The listing builds one solid part. Answer for the finished solid, in the listing's coordinates (mm). Face numbers are marked on the shaded views. A direction names the side the tool comes from. Give positions to 0.01 mm unless a question says otherwise; leave off trailing zeros. Order: outer loops, then holes, each group sorted by start corner. A loop starts at its lowest first (then second) coordinate and runs counter-clockwise, first axis right, second up. Notation, with made-up numbers: (58.5, 87.5) - (83.5, 87.5) arc R11 cw to (83.5, 108.5) - close; hole circle Ø11 at (48.25, 82.5). An arc over 180 degrees is marked (long way). Write each question's results on one line, items separated by ' | '. Start each with the question number.
1. A flat-ended cylindrical pin translates along its axis: pin 1 (15 mm diameter, centred on x = 22.225, y = 38.1, fed in from -Z). Find the tip coordinate at first contact, or state that the pin passes through.
2. Section C-C (z = 10) is taken. Give the vertices of the cut face in (x, y) (1 decimal), and give its area (3 significant figures).
3. Determine the mould class of the marked faces 1, 2, 3 and 4 for opening direction X: released by +X, released by -X, zero draft, split by the parting line, or undercut.
4. Find the intervals of material crossed by L1, parallel to Y at x = -70.5, z = 3; L2, parallel to X at y = -90, z = 6.5; L3, parallel to Y at x = 44, z = 42.5, in increasing order.
5. Section A-A (y = 38.1) is taken. State how many separate pieces and enclosed holes the cut face has, and give its area (3 significant figures).
6. Which of the six approach directions +Z, -Z, +X, -X, +Y, -Y give full straight-line access (tool end or side, diameter ignored) to the marked faces 5 and 6?
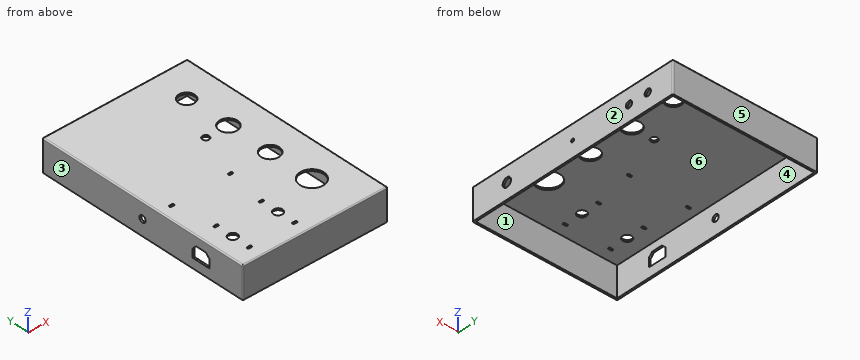
from build123d import *

# Parameters (mm, degrees)
F0_W      = 203.2
F0_H      = 304.8
F1_DEPTH  = 44.45
F2_T      = -2.54
F3_W      = 6.35
F3_H      = 3.175
F4_DEPTH  = 25.4
F5_R      = 1.58749
F7_D      = 33.3375
F7_DEPTH  = 19.05
F7_TIP    = 10.0155954434
F8_D      = 25.4
F8_DEPTH  = 19.05
F8_TIP    = 7.6309298617
F9_D      = 22.225
F9_DEPTH  = 19.05
F9_TIP    = 6.6770636289
F11_D     = 4.7625
F11_DEPTH = 19.05
F11_TIP   = 1.4307993491
F12_D     = 9.525
F12_DEPTH = 19.05
F12_TIP   = 2.8615986981
F13_D     = 12.7
F13_DEPTH = 19.05
F13_TIP   = 3.8154649308
F15_DEPTH = 25.4
F16_D     = 12.7
F16_DEPTH = 19.05
F16_TIP   = 3.8154649308
F17_W     = 6.35
F17_H     = 3.175
F18_DEPTH = 25.4
F19_R     = 1.58749
F20_D     = 9.525
F20_DEPTH = 5.715
F20_TIP   = 2.8615986981
F21_D     = 9.525
F21_DEPTH = 5.715
F21_TIP   = 2.8615986981
F22_R     = 1.5875


# Not quite as in the source:
# - a fillet or chamfer is up to 0.001 mm smaller than in the source, because OpenCascade refuses the exact size


with BuildPart() as f1:
    # F0 (on Top) → F1 (new body)
    with BuildSketch(Plane.XY):
        Rectangle(F0_W, F0_H)
    extrude(amount=F1_DEPTH)

    # F2
    f2_openings = [f1.faces().sort_by_distance(p)[0] for p in [
        (0, 0, 0),
    ]]
    offset(amount=F2_T, openings=f2_openings)

    # F3 (on face) → F4 (cut)
    with BuildSketch(Plane.XY.offset(44.45)):
        with Locations((-74.6125, -133.35)):
            Rectangle(F3_W, F3_H)
        with Locations((-74.6125, -82.55)):
            Rectangle(F3_W, F3_H)
        with Locations((-11.1125, -82.55)):
            Rectangle(F3_W, F3_H)
        with Locations((-11.1125, -133.35)):
            Rectangle(F3_W, F3_H)
    extrude(amount=-F4_DEPTH, mode=Mode.SUBTRACT)

    # F5 (radius 1.5875 in the source; OpenCascade refuses exactly that, so slightly less here)
    f5_edges = [f1.edges().sort_by_distance(p)[0] for p in [
        (-77.7875, -131.7625, 43.18),
        (-14.2875, -131.7625, 43.18),
        (-77.7875, -80.9625, 43.18),
        (-71.4375, -80.9625, 43.18),
        (-7.9375, -80.9625, 43.18),
        (-7.9375, -131.7625, 43.18),
        (-71.4375, -131.7625, 43.18),
        (-14.2875, -134.9375, 43.18),
        (-77.7875, -134.9375, 43.18),
        (-77.7875, -84.1375, 43.18),
        (-14.2875, -84.1375, 43.18),
        (-7.9375, -134.9375, 43.18),
        (-7.9375, -84.1375, 43.18),
        (-71.4375, -84.1375, 43.18),
        (-71.4375, -134.9375, 43.18),
        (-14.2875, -80.9625, 43.18),
    ]]
    fillet(f5_edges, radius=F5_R)

    # F7
    with Locations(Plane.XY.offset(44.45)):
        with Locations((53.975, -88.9)):
            Hole(F7_D / 2, depth=F7_DEPTH)
            with Locations((0, 0, -(F7_DEPTH + F7_TIP / 2))):  # 118° drill point
                Cone(0, F7_D / 2, F7_TIP, mode=Mode.SUBTRACT)

    # F8
    with Locations(Plane.XY.offset(44.45)):
        with Locations((53.975, -25.4), (53.975, 38.1)):
            Hole(F8_D / 2, depth=F8_DEPTH)
            with Locations((0, 0, -(F8_DEPTH + F8_TIP / 2))):  # 118° drill point
                Cone(0, F8_D / 2, F8_TIP, mode=Mode.SUBTRACT)

    # F9
    with Locations(Plane.XY.offset(44.45)):
        with Locations((53.975, 101.6)):
            Hole(F9_D / 2, depth=F9_DEPTH)
            with Locations((0, 0, -(F9_DEPTH + F9_TIP / 2))):  # 118° drill point
                Cone(0, F9_D / 2, F9_TIP, mode=Mode.SUBTRACT)

    # F11
    with Locations(Plane.YZ.offset(101.6)):
        with Locations((0, 22.225)):
            Hole(F11_D / 2, depth=F11_DEPTH)
            with Locations((0, 0, -(F11_DEPTH + F11_TIP / 2))):  # 118° drill point
                Cone(0, F11_D / 2, F11_TIP, mode=Mode.SUBTRACT)

    # F12
    with Locations(Plane.YZ.offset(101.6)):
        with Locations((85.725, 22.225), (114.3, 22.225)):
            Hole(F12_D / 2, depth=F12_DEPTH)
            with Locations((0, 0, -(F12_DEPTH + F12_TIP / 2))):  # 118° drill point
                Cone(0, F12_D / 2, F12_TIP, mode=Mode.SUBTRACT)

    # F13
    with Locations(Plane.YZ.offset(101.6)):
        with Locations((-100.0125, 22.225)):
            Hole(F13_D / 2, depth=F13_DEPTH)
            with Locations((0, 0, -(F13_DEPTH + F13_TIP / 2))):  # 118° drill point
                Cone(0, F13_D / 2, F13_TIP, mode=Mode.SUBTRACT)

    # F14 (on face) → F15 (cut)
    with BuildSketch(Plane(origin=(-101.6, 0, 0), x_dir=(0, -1, 0), z_dir=(-1, 0, 0))):
        Polygon((101.6, 25.5999010921), (96.2436510921, 30.95625), (81.5563489079, 30.95625), (76.2, 25.5999010921), (76.2, 18.8500989079), (81.5563489079, 13.49375), (96.2436510921, 13.49375), (101.6, 18.8500989079), align=None)
        Polygon((81.5563489079, 13.49375), (76.2, 18.8500989079), (76.2, 13.49375), align=None)
        Polygon((101.6, 13.49375), (101.6, 18.8500989079), (96.2436510921, 13.49375), align=None)
    extrude(amount=-F15_DEPTH, mode=Mode.SUBTRACT)

    # F16
    with Locations(Plane.XY.offset(44.45)):
        with Locations((-74.6125, -107.95), (-11.1125, -107.95)):
            Hole(F16_D / 2, depth=F16_DEPTH)
            with Locations((0, 0, -(F16_DEPTH + F16_TIP / 2))):  # 118° drill point
                Cone(0, F16_D / 2, F16_TIP, mode=Mode.SUBTRACT)

    # F17 (on face) → F18 (cut)
    with BuildSketch(Plane.XY.offset(44.45)):
        with Locations((-84.1375, -25.4)):
            Rectangle(F17_W, F17_H)
        with Locations((-1.5875, -25.4)):
            Rectangle(F17_W, F17_H)
    extrude(amount=-F18_DEPTH, mode=Mode.SUBTRACT)

    # F19 (radius 1.5875 in the source; OpenCascade refuses exactly that, so slightly less here)
    f19_edges = [f1.edges().sort_by_distance(p)[0] for p in [
        (-87.3125, -23.8125, 43.18),
        (-4.7625, -23.8125, 43.18),
        (-80.9625, -23.8125, 43.18),
        (1.5875, -23.8125, 43.18),
        (-87.3125, -26.9875, 43.18),
        (-4.7625, -26.9875, 43.18),
        (-80.9625, -26.9875, 43.18),
        (1.5875, -26.9875, 43.18),
    ]]
    fillet(f19_edges, radius=F19_R)

    # F20
    with Locations(Plane(origin=(-101.6, 0, 0), x_dir=(0, -1, 0), z_dir=(-1, 0, 0))):
        with Locations((0, 22.225)):
            Hole(F20_D / 2, depth=F20_DEPTH)
            with Locations((0, 0, -(F20_DEPTH + F20_TIP / 2))):  # 118° drill point
                Cone(0, F20_D / 2, F20_TIP, mode=Mode.SUBTRACT)

    # F21
    with Locations(Plane.XY.offset(44.45)):
        with Locations((22.225, 38.1)):
            Hole(F21_D / 2, depth=F21_DEPTH)
            with Locations((0, 0, -(F21_DEPTH + F21_TIP / 2))):  # 118° drill point
                Cone(0, F21_D / 2, F21_TIP, mode=Mode.SUBTRACT)

    # F22
    f22_edges = [f1.edges().sort_by_distance(p)[0] for p in [
        (0, -152.4, 44.45),
        (101.6, 0, 44.45),
        (101.6, -152.4, 22.225),
        (0, 152.4, 44.45),
        (101.6, 152.4, 22.225),
        (-101.6, 152.4, 22.225),
        (-101.6, 0, 44.45),
        (-101.6, -152.4, 22.225),
    ]]
    fillet(f22_edges, radius=F22_R)


solid = f1.part
Reported:
1) pin 1: z = 41.91
2) outline: (-101.6, -150.8) arc R1.6 ccw to (-100, -152.4) - (100, -152.4) arc R1.6 ccw to (101.6, -150.8) - (101.6, 150.8) arc R1.6 ccw to (100, 152.4) - (-100, 152.4) arc R1.6 ccw to (-101.6, 150.8) - close; hole (-99.1, -149.9) - (99.1, -149.9) - (99.1, 149.9) - (-99.1, 149.9) - close | area: 2,550 mm²
3) face 1: undercut | face 2: released by +X | face 3: released by -X | face 4: undercut
4) L1: -152.4 to -149.86, 149.86 to 152.4 | L2: -101.6 to -99.06, 99.06 to 101.6 | L3: -152.4 to -102.25, -75.55 to -33.26, -17.54 to 30.24, 45.96 to 96.7, 106.5 to 152.4
5) separate pieces: 3 | enclosed holes: 0 | area: 639 mm²
6) face 5: +Z, -Z, +X, -X, +Y | face 6: -Z
